Build history of the part. All positions in model axes, mm. A direction names the side the tool comes from. Give positions to 0.01 mm unless a question says otherwise; leave off trailing zeros. Order: outer loops, then holes, each group sorted by start corner. A loop starts at its lowest first (then second) coordinate and runs counter-clockwise, first axis right, second up. Notation, with made-up numbers: (89.5, 80.25) -> (128.5, 80.25) arc R19 cw to (128.5, 97.25) -> close; hole circle Ø4 at (-6.5, 62). An arc over 180 degrees is marked (long way). One line per item, written item: value. Start each with the question number.
(1) Two-plate mould, pull along X, no slides. Class faces 1 (the flat face through (-47, -2, 51.588)), 2 (the flat face through (-120.65, -2, 82)), 3 (the flat face through (-84.525, -2, 62)), 4 (the flat face through (12.7, -2, 22)): +X half, -X half, draft (parallel to the pull), parting line (faces both ways), or undercut.
(2) Saw through at A-A on x = -166. Give the cut face in (y, z), plus the area to 3 significant figures.
(3) Which spindle directions (+Z, -Z, +X, -X, +Y, -Y) get a long thin tool onto all of the face, cutting with end or side? Do faces 5 (the flat face through (-114, -2, 4.762)), 6 (the flat face through (-267, -2, 80)), 7 (the flat face through (-29.763, -2, 42)), 8 (the flat face through (-2, -2, 37.938)). Say none if no direction does.
(4) Probe line 1 (X direction, y = -0.45, z = 64) (3 decimals); line 2 (X direction, y = -3.8, z = 21); line 3 (X direction, y = -4.55, z = 78). List the from-to ranges inside material, lowest first.
(5) Pin check, flat tips, straight feed: pin 1 (2.5 mm diameter, centred on y = -2.5, z = 62, fed in from +X) (3 decimals); pin 2 (0.9 mm diameter, centred on x = -78, y = -2.5, fed in from +Z); pin 3 (1 mm diameter, centred on y = -3.5, z = 34.5, fed in from +X). Stop position of each tip, or through.
```python
from build123d import *

# Parameters (mm, degrees)
F1_DEPTH  = 4.7625
F2_W      = 19.05
F2_H      = 4.7625
F2_W_2    = 25.4
F3_DEPTH  = 25.4
F4_W      = 4.7625
F4_H      = 6.825
F4_W_2    = 0.2375
F4_W_3    = 4.525
F5_DEPTH  = 25.4
F6_W      = 31.75
F6_H      = 24.7625
F7_DEPTH  = 4.7625
F8_W      = 4.7625
F8_H      = 6.825
F9_DEPTH  = 25.4
F10_W     = 6.35
F10_H     = 4.7625
F11_DEPTH = 25.4
F12_W     = 10
F12_H     = 4.7625
F13_DEPTH = 25.4
F14_W     = 25.4
F14_H     = 4.7625
F14_W_2   = 26.3625
F15_DEPTH = 25.4
F17_DEPTH = 25.4


with BuildPart() as f1:
    # F0 (on Front) → F1 (new body)
    with BuildSketch(Plane.XZ):
        Polygon((-273.05, 0), (0, 0), (0, 44.7625), (-44.7625, 44.7625), (-44.7625, 64.7625), (-89.525, 64.7625), (-89.525, 84.7625), (-129.525, 84.7625), (-273.05, 84.7625), align=None)
    extrude(amount=F1_DEPTH)

    # F2 (on face) → F3 (cut)
    with BuildSketch(Plane.XZ.offset(4.7625)):
        with Locations((-263.525, 2.38125)):
            Rectangle(F2_W, F2_H)
        with Locations((-12.7, 2.38125)):
            Rectangle(F2_W_2, F2_H)
        with Locations((-63.5, 2.38125)):
            Rectangle(F2_W_2, F2_H)
        with Locations((-114.3, 2.38125)):
            Rectangle(F2_W_2, F2_H)
        with Locations((-165.1, 2.38125)):
            Rectangle(F2_W_2, F2_H)
        with Locations((-215.9, 2.38125)):
            Rectangle(F2_W_2, F2_H)
    extrude(amount=-F3_DEPTH, mode=Mode.SUBTRACT)

    # F4 (on face) → F5 (cut)
    with BuildSketch(Plane.XZ.offset(4.7625)):
        with Locations((-47.14375, 61.35)):
            Rectangle(F4_W, F4_H)
        with Locations((-44.88125, 48.175)):
            Rectangle(F4_W_2, F4_H)
        with Locations((-47.2625, 48.175)):
            Rectangle(F4_W_3, F4_H)
        with Locations((-91.90625, 81.35)):
            Rectangle(F4_W, F4_H)
        with Locations((-91.90625, 68.175)):
            Rectangle(F4_W, F4_H)
    extrude(amount=-F5_DEPTH, mode=Mode.SUBTRACT)

    # F6 (on face) → F7 (join)
    with BuildSketch(Plane.XZ.offset(4.7625)):
        with Locations((15.875, 12.38125)):
            Rectangle(F6_W, F6_H)
    extrude(amount=-F7_DEPTH)

    # F8 (on face) → F9 (cut)
    with BuildSketch(Plane.XZ.offset(4.7625)):
        with Locations((-2.38125, 41.35)):
            Rectangle(F8_W, F8_H)
        with Locations((-2.38125, 28.175)):
            Rectangle(F8_W, F8_H)
    extrude(amount=-F9_DEPTH, mode=Mode.SUBTRACT)

    # F10 (on face) → F11 (cut)
    with BuildSketch(Plane.XZ.offset(4.7625)):
        with Locations((9.525, 22.38125)):
            Rectangle(F10_W, F10_H)
        with Locations((22.225, 22.38125)):
            Rectangle(F10_W, F10_H)
    extrude(amount=-F11_DEPTH, mode=Mode.SUBTRACT)

    # F12 (on face) → F13 (cut)
    with BuildSketch(Plane.XZ.offset(4.7625)):
        with Locations((-34.7625, 42.38125)):
            Rectangle(F12_W, F12_H)
        with Locations((-14.7625, 42.38125)):
            Rectangle(F12_W, F12_H)
        with Locations((-79.525, 62.38125)):
            Rectangle(F12_W, F12_H)
        with Locations((-59.525, 62.38125)):
            Rectangle(F12_W, F12_H)
    extrude(amount=-F13_DEPTH, mode=Mode.SUBTRACT)

    # F14 (on face) → F15 (cut)
    with BuildSketch(Plane.XZ.offset(4.7625)):
        with Locations((-209.55, 82.38125)):
            Rectangle(F14_W, F14_H)
        with Locations((-260.35, 82.38125)):
            Rectangle(F14_W, F14_H)
        with Locations((-158.75, 82.38125)):
            Rectangle(F14_W, F14_H)
        with Locations((-107.46875, 82.38125)):
            Rectangle(F14_W_2, F14_H)
    extrude(amount=-F15_DEPTH, mode=Mode.SUBTRACT)

    # F16 (on face) → F17 (cut)
    with BuildSketch(Plane.XZ.offset(4.7625)):
        Polygon((-33.6625, 40), (-35.8625, 40), (-35.8625, 36), (-36.9625, 36), (-36.9625, 34), (-35.8625, 34), (-35.8625, 30.7625), (-34.7625, 30.7625), (-33.6625, 30.7625), (-33.6625, 34), (-32.5625, 34), (-32.5625, 36), (-33.6625, 36), align=None)
        Polygon((-13.6625, 40), (-15.8625, 40), (-15.8625, 36), (-16.9625, 36), (-16.9625, 34), (-15.8625, 34), (-15.8625, 30.7625), (-14.7625, 30.7625), (-13.6625, 30.7625), (-13.6625, 34), (-12.5625, 34), (-12.5625, 36), (-13.6625, 36), align=None)
        Polygon((-78.425, 60), (-80.625, 60), (-80.625, 56), (-81.725, 56), (-81.725, 54), (-80.625, 54), (-80.625, 50.7625), (-79.525, 50.7625), (-78.425, 50.7625), (-78.425, 54), (-77.325, 54), (-77.325, 56), (-78.425, 56), align=None)
        Polygon((-58.425, 60), (-60.625, 60), (-60.625, 56), (-61.725, 56), (-61.725, 54), (-60.625, 54), (-60.625, 50.7625), (-59.525, 50.7625), (-58.425, 50.7625), (-58.425, 54), (-57.325, 54), (-57.325, 56), (-58.425, 56), align=None)
        Polygon((-157.65, 80), (-159.85, 80), (-159.85, 76), (-160.95, 76), (-160.95, 74), (-159.85, 74), (-159.85, 70.7625), (-158.75, 70.7625), (-157.65, 70.7625), (-157.65, 74), (-156.55, 74), (-156.55, 76), (-157.65, 76), align=None)
        Polygon((-208.45, 80), (-210.65, 80), (-210.65, 76), (-211.75, 76), (-211.75, 74), (-210.65, 74), (-210.65, 70.7625), (-209.55, 70.7625), (-208.45, 70.7625), (-208.45, 74), (-207.35, 74), (-207.35, 76), (-208.45, 76), align=None)
        Polygon((-259.25, 80), (-261.45, 80), (-261.45, 76), (-262.55, 76), (-262.55, 74), (-261.45, 74), (-261.45, 70.7625), (-260.35, 70.7625), (-259.25, 70.7625), (-259.25, 74), (-258.15, 74), (-258.15, 76), (-259.25, 76), align=None)
        Polygon((-106.85, 80), (-109.05, 80), (-109.05, 76), (-110.15, 76), (-110.15, 74), (-109.05, 74), (-109.05, 70.7625), (-107.95, 70.7625), (-106.85, 70.7625), (-106.85, 74), (-105.75, 74), (-105.75, 76), (-106.85, 76), align=None)
    extrude(amount=-F17_DEPTH, mode=Mode.SUBTRACT)


solid = f1.part
```
Results below:
1. face 1: draft
1. face 2: +X half
1. face 3: undercut
1. face 4: undercut
2. outline: (-4.76, 4.76) -> (0, 4.76) -> (0, 80) -> (-4.76, 80) -> close
2. area: 358 mm²
3. face 5: -Z, +Y, -Y
3. face 6: +Z, -X, +Y, -Y
3. face 7: +Z, +Y, -Y
3. face 8: +Z, +X, +Y, -Y
4. line 1: x = -273.05 to -84.525, -74.525 to -64.525, -54.525 to -49.525
4. line 2: x = -273.05 to 6.35, 12.7 to 19.05, 25.4 to 31.75
4. line 3: x = -273.05 to -261.45, -259.25 to -210.65, -208.45 to -159.85, -157.65 to -109.05, -106.85 to -94.29
5. pin 1: stops at x = -49.525
5. pin 2: stops at z = 60
5. pin 3: stops at x = 0
